```python
from build123d import *

# Parameters (mm, degrees)
CROQUIS1_W              = 70
CROQUIS1_H              = 105
SALIENTE_EXTRUIR1_DEPTH = 3.175
CROQUIS2_R              = 16.5
SALIENTE_EXTRUIR2_DEPTH = 3.175
CROQUIS3_W              = 26
CROQUIS3_H              = 6
CORTAR_EXTRUIR1_DEPTH   = 3.175
CROQUIS4_W              = 3
CROQUIS4_H              = 11
CORTAR_EXTRUIR2_DEPTH   = 1


with BuildPart() as part:
    # Croquis1 → Saliente-Extruir1 (new body)
    with BuildSketch(Plane.XY):
        with Locations((35, -52.5)):
            Rectangle(CROQUIS1_W, CROQUIS1_H)
    extrude(amount=SALIENTE_EXTRUIR1_DEPTH)

    # Croquis2 → Saliente-Extruir2 (add)
    with BuildSketch(Plane.XY.offset(3.175)):
        with Locations((35, -26.25)):
            Circle(CROQUIS2_R)
        with Locations((35, -78.75)):
            Circle(CROQUIS2_R)
    extrude(amount=SALIENTE_EXTRUIR2_DEPTH)

    # Croquis3 → Cortar-Extruir1 (cut)
    with BuildSketch(Plane.XY.offset(6.35)):
        with Locations((35, -9.75)):
            Rectangle(CROQUIS3_W, CROQUIS3_H)
        with Locations((35, -42.75)):
            Rectangle(CROQUIS3_W, CROQUIS3_H)
        with Locations((35, -62.25)):
            Rectangle(CROQUIS3_W, CROQUIS3_H)
        with Locations((35, -95.25)):
            Rectangle(CROQUIS3_W, CROQUIS3_H)
    extrude(amount=-CORTAR_EXTRUIR1_DEPTH, mode=Mode.SUBTRACT)

    # Croquis4 → Cortar-Extruir2 (cut)
    with BuildSketch(Plane.XY.offset(6.35)):
        with Locations((27.5, -29.25)):
            Rectangle(CROQUIS4_W, CROQUIS4_H)
        with Locations((42.5, -29.25)):
            Rectangle(CROQUIS4_W, CROQUIS4_H)
        with BuildLine():
            Line((34.632057675, -19.532945654), (35.367942325, -19.532945654))
            ThreePointArc((35.367942325, -19.532945654), (36.923577244, -18.888580572), (37.567942325, -17.332945654))
            Line((37.567942325, -17.332945654), (37.567942325, -14.967054346))
            Line((37.567942325, -14.967054346), (32.432057675, -14.967054346))
            Line((32.432057675, -14.967054346), (32.432057675, -17.332945654))
            ThreePointArc((32.432057675, -17.332945654), (33.076422756, -18.888580572), (34.632057675, -19.532945654))
        make_face()
        with Locations((42.5, -81.75)):
            Rectangle(CROQUIS4_W, CROQUIS4_H)
        with Locations((27.5, -81.75)):
            Rectangle(CROQUIS4_W, CROQUIS4_H)
        with BuildLine():
            Line((34.632057675, -71.973579429), (35.367942325, -71.973579429))
            ThreePointArc((35.367942325, -71.973579429), (36.923577244, -71.329214348), (37.567942325, -69.773579429))
            Line((37.567942325, -69.773579429), (37.567942325, -67.526420571))
            Line((37.567942325, -67.526420571), (32.432057675, -67.526420571))
            Line((32.432057675, -67.526420571), (32.432057675, -69.773579429))
            ThreePointArc((32.432057675, -69.773579429), (33.076422756, -71.329214348), (34.632057675, -71.973579429))
        make_face()
    extrude(amount=-CORTAR_EXTRUIR2_DEPTH, mode=Mode.SUBTRACT)


solid = part.part
```
The model under review builds one solid part; all positions refer to its coordinate system, in mm. A direction names the side the tool comes from. Round coordinates to 2 decimals unless told otherwise and drop trailing zeros. Write each loop counter-clockwise with the first axis right and the second up, starting at its lowest first coordinate (ties: lowest second). Pieces come first, ordered by that corner, then holes. Notation, with made-up numbers: M 14,83 L 24,83 A28 cw 24,104 Z; hole C 76.25,53.25 d5. An arc over 180 degrees is marked long. Use CSV: the item, a comma, the result in double quotes. Start each with the question number.
(1) Tool access review of faces 1 (the face through (18.5, -78.5, 4.7)), 2 (the face through (51.5, -79, 4.7)), 3 (the face through (27, -82, 5.35)), 4 (the face through (35, -79, 6.35)), 5 (the face through (35, -12.75, 5)): name each direction out of +Z, -Z, +X, -X, +Y, -Y from which nothing blocks a thin tool from reaching the whole face with its end or side.
(2) We need section B-B, the plane y = -95. State the section outline as (x, z) points (3 decimals), then the cut area to 3 significant figures.
(3) For line 1 along Z through (x, y) = (9, -16.5) (3 decimals); line 2 along Z through (x, y) = (34, -15); line 3 along X through (y, z) = (-90.5, 4.25), list the stretches that pass through material, from the lowest coordinate up.
(4) Clearance check with flat-ended pins moving along their axes: P1, Ø0.5, axis at x = 42, z = 6, coming from the -Y side; P2, Ø0.5, axis at x = 27, z = 5.5, coming from the +Y side; P3, Ø1.1, axis at y = -84, z = 6, coming from the -X side; P4, Ø3, axis at x = 54, z = 5, coming from the -Y side. State where each tip first meets the part, or that it passes through.
(5) We need section D-D, the plane y = -82. State the section outline as (x, z) points (3 decimals).
(6) We need section A-A, the plane x = 46. State the section outline as (y, z) points (3 decimals).
(7) The part is to be moulded in two halves that separate along X. For faces 6 (the face through (51.5, -26.5, 4.7)), 7 (the face through (33.06, -18.87, 5.86)), 8 (the face through (18.5, -26, 4.7)), say which applies: +X half, -X half, draft (parallel to the pull), parting line (faces both ways), or undercut.
(8) We need section C-C, the plane x = 23. State the section outline as (y, z) points (3 decimals).
Findings:
1,face 1,"+Z, -X"
1,face 2,"+Z, +X"
1,face 3,"+Z"
1,face 4,"+Z, +X, -X, +Y, -Y"
1,face 5,"+Z, +X, -X, +Y"
2,outline,"M 0,0 L 70,0 L 70,3.175 L 0,3.175 Z"
2,area,"222 mm^2"
3,line 1,"0 to 3.175"
3,line 2,"0 to 5.35"
3,line 3,"23.42 to 46.58"
4,P1,"y = -92.25"
4,P2,"y = -12.75"
4,P3,"x = 19.18"
4,P4,"through"
5,outline,"M 0,0 L 70,0 L 70,3.175 L 51.177,3.175 L 51.177,6.35 L 44,6.35 L 44,5.35 L 41,5.35 L 41,6.35 L 29,6.35 L 29,5.35 L 26,5.35 L 26,6.35 L 18.823,6.35 L 18.823,3.175 L 0,3.175 Z"
6,outline,"M -105,0 L 0,0 L 0,3.175 L -13.952,3.175 L -13.952,6.35 L -38.548,6.35 L -38.548,3.175 L -66.452,3.175 L -66.452,6.35 L -91.048,6.35 L -91.048,3.175 L -105,3.175 Z"
7,face 6,"+X half"
7,face 7,"undercut"
7,face 8,"-X half"
8,outline,"M -105,0 L 0,0 L 0,3.175 L -14.925,3.175 L -14.925,6.35 L -37.575,6.35 L -37.575,3.175 L -67.425,3.175 L -67.425,6.35 L -90.075,6.35 L -90.075,3.175 L -105,3.175 Z"
